Model file for the job. Use its own axes, mm. A direction names the side the tool comes from. Round coordinates to 2 decimals unless told otherwise and drop trailing zeros. Loops run counter-clockwise (first coordinate to the right, second up) from the corner with the lowest first, then second, coordinate; pieces in that order, holes last. Notation, with made-up numbers: (-17.75, 54) - (29.25, 54) arc R5 cw to (29.25, 63) - close; hole circle Ø3 at (25, -17.5). An arc over 180 degrees is marked (long way). Answer as a JSON object with one key per item and string values.
from build123d import *

# Parameters (mm, degrees)
SKETCH1_W           = 457.2
SKETCH1_H           = 457.2
BOSS_EXTRUDE1_DEPTH = 3
SKETCH2_R           = 1.875
CUT_EXTRUDE2_DEPTH  = 324.303139484
SKETCH3_R           = 1.625
CUT_EXTRUDE3_DEPTH  = 324.303139484
CUT_EXTRUDE4_DEPTH  = 324.303139484
SKETCH5_W           = 250
SKETCH5_H           = 250
CUT_EXTRUDE5_DEPTH  = 324.303139484


with BuildPart() as part:
    # Sketch1 → Boss-Extrude1 (new body)
    with BuildSketch(Plane(origin=(0, 0, 0), x_dir=(1, 0, 0), z_dir=(0, 1, 0))):
        Rectangle(SKETCH1_W, SKETCH1_H)
    extrude(amount=BOSS_EXTRUDE1_DEPTH)

    # Sketch2 → Cut-Extrude2 (cut, through all)
    with BuildSketch(Plane(origin=(0, 3, 0), x_dir=(1, 0, 0), z_dir=(0, 1, 0))):
        with Locations(Location((-173.2, 203.2, 0), (0, 0, 90))):
            Circle(SKETCH2_R)
        with Locations(Location((173.2, 203.2, 0), (0, 0, 270))):
            Circle(SKETCH2_R)
        with Locations(Location((-173.2, -203.2, 0), (0, 0, 270))):
            Circle(SKETCH2_R)
        with Locations(Location((-203.2, 203.2, 0), (0, 0, 270))):
            Circle(SKETCH2_R)
        with Locations(Location((-203.2, 179.2, 0), (0, 0, 270))):
            Circle(SKETCH2_R)
        with Locations(Location((-173.2, 179.2, 0), (0, 0, 270))):
            Circle(SKETCH2_R)
        with Locations(Location((-173.2, -179.2, 0), (0, 0, 90))):
            Circle(SKETCH2_R)
        with Locations(Location((-203.2, -179.2, 0), (0, 0, 90))):
            Circle(SKETCH2_R)
        with Locations(Location((-203.2, -203.2, 0), (0, 0, 90))):
            Circle(SKETCH2_R)
        with Locations(Location((173.2, 179.2, 0), (0, 0, 90))):
            Circle(SKETCH2_R)
        with Locations(Location((203.2, 179.2, 0), (0, 0, 90))):
            Circle(SKETCH2_R)
        with Locations(Location((203.2, 203.2, 0), (0, 0, 90))):
            Circle(SKETCH2_R)
        with Locations(Location((203.2, -203.2, 0), (0, 0, 270))):
            Circle(SKETCH2_R)
        with Locations(Location((203.2, -179.2, 0), (0, 0, 270))):
            Circle(SKETCH2_R)
        with Locations(Location((173.2, -179.2, 0), (0, 0, 270))):
            Circle(SKETCH2_R)
        with Locations(Location((173.2, -203.2, 0), (0, 0, 90))):
            Circle(SKETCH2_R)
    extrude(amount=-CUT_EXTRUDE2_DEPTH, mode=Mode.SUBTRACT)

    # Sketch3 → Cut-Extrude3 (cut, through all)
    with BuildSketch(Plane(origin=(0, 3, 0), x_dir=(1, 0, 0), z_dir=(0, 1, 0))):
        with Locations(Location((-188.2, 191.2, 0), (0, 0, 270))):
            Circle(SKETCH3_R)
        with Locations(Location((-188.2, -191.2, 0), (0, 0, 90))):
            Circle(SKETCH3_R)
        with Locations(Location((188.2, 191.2, 0), (0, 0, 90))):
            Circle(SKETCH3_R)
        with Locations(Location((188.2, -191.2, 0), (0, 0, 270))):
            Circle(SKETCH3_R)
        with Locations(Location((-188.2, 0, 0), (0, 0, 270))):
            Circle(SKETCH3_R)
        with Locations(Location((188.2, 0, 0), (0, 0, 90))):
            Circle(SKETCH3_R)
    extrude(amount=-CUT_EXTRUDE3_DEPTH, mode=Mode.SUBTRACT)

    # Sketch4 → Cut-Extrude4 (cut, through all)
    with BuildSketch(Plane(origin=(0, 3, 0), x_dir=(1, 0, 0), z_dir=(0, 1, 0))):
        with BuildLine():
            Line((-200.7, 131.2), (-200.7, 51.2))
            ThreePointArc((-200.7, 51.2), (-188.2, 38.7), (-175.7, 51.2))
            Line((-175.7, 51.2), (-175.7, 131.2))
            ThreePointArc((-175.7, 131.2), (-188.2, 143.7), (-200.7, 131.2))
        make_face()
        with BuildLine():
            Line((-175.7, -131.2), (-175.7, -51.2))
            ThreePointArc((-175.7, -51.2), (-188.2, -38.7), (-200.7, -51.2))
            Line((-200.7, -51.2), (-200.7, -131.2))
            ThreePointArc((-200.7, -131.2), (-188.2, -143.7), (-175.7, -131.2))
        make_face()
        with BuildLine():
            Line((200.7, -131.2), (200.7, -51.2))
            ThreePointArc((200.7, -51.2), (188.2, -38.7), (175.7, -51.2))
            Line((175.7, -51.2), (175.7, -131.2))
            ThreePointArc((175.7, -131.2), (188.2, -143.7), (200.7, -131.2))
        make_face()
        with BuildLine():
            Line((175.7, 131.2), (175.7, 51.2))
            ThreePointArc((175.7, 51.2), (188.2, 38.7), (200.7, 51.2))
            Line((200.7, 51.2), (200.7, 131.2))
            ThreePointArc((200.7, 131.2), (188.2, 143.7), (175.7, 131.2))
        make_face()
    extrude(amount=-CUT_EXTRUDE4_DEPTH, mode=Mode.SUBTRACT)

    # Sketch5 → Cut-Extrude5 (cut, through all)
    with BuildSketch(Plane(origin=(0, 3, 0), x_dir=(1, 0, 0), z_dir=(0, 1, 0))):
        Rectangle(SKETCH5_W, SKETCH5_H)
    extrude(amount=-CUT_EXTRUDE5_DEPTH, mode=Mode.SUBTRACT)


solid = part.part
1) Slice it at B-B on y = 1.9. Count the separate pieces of the cut face and the enclosed holes in it, then the cut area to 3 significant figures.
Values follow:
{"separate pieces": "1", "enclosed holes": "27", "area": "136,000 mm²"}
2) Drop a flat-ended pin along its axis: P1, Ø3, axis at x = 173.2, z = -179.2, coming from the +Y side. Give the stop position or say it passes through.
Values follow:
{"P1": "through"}
3) Tool access for faces 3 (the flat face through (-156, 3, -3)), 4 (the cylindrical face through (187.925, 1.521, 143.697)): list every direction of +Z, -Z, +X, -X, +Y, -Y with a clear straight run to the whole face (end or side of a thin tool).
Values follow:
{"face 3": "+Z, -Z, +X, -X, +Y", "face 4": "+Y, -Y"}
4) Two-plate mould, pull along Z, no slides. Class faces 1 (the flat face through (-156, 0, -3)), 2 (the cylindrical face through (-188.475, 1.521, -38.703)): pulls with the +Z half, pulls with the -Z half, needs draft (parallel to the pull), parting line crosses it, or undercut.
Values follow:
{"face 1": "needs draft", "face 2": "undercut"}
5) Slice it at A-A on z = 99. List the corners of the cut face in (x, y), then the cut area to 3 significant figures.
Values follow:
{"outline": "(-228.6, 0) - (-200.7, 0) - (-200.7, 3) - (-228.6, 3) - close; (-175.7, 0) - (-125, 0) - (-125, 3) - (-175.7, 3) - close; (125, 0) - (175.7, 0) - (175.7, 3) - (125, 3) - close; (200.7, 0) - (228.6, 0) - (228.6, 3) - (200.7, 3) - close", "area": "472 mm²"}
6) Probe probe 1 along X at (y, z) = (1.9, 179.2) (3 decimals); probe 2 along X at (y, z) = (1.4, 64.5); probe 3 along Z at (x, y) = (-173.2, 2.05) (3 decimals). List the from-to ranges inside material, lowest first.
Values follow:
{"probe 1": "-228.6 to -205.075, -201.325 to -175.075, -171.325 to 171.325, 175.075 to 201.325, 205.075 to 228.6", "probe 2": "-228.6 to -200.7, -175.7 to -125, 125 to 175.7, 200.7 to 228.6", "probe 3": "-228.6 to -205.075, -201.325 to -181.075, -177.325 to 177.325, 181.075 to 201.325, 205.075 to 228.6"}
